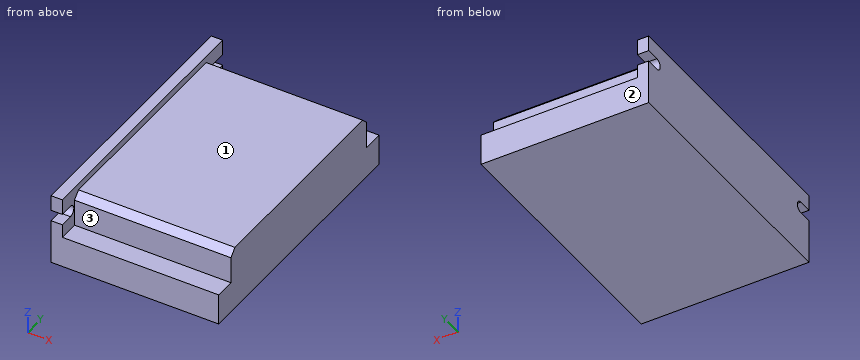
from build123d import *

# Parameters (mm, degrees)
SKETCH_1_W          = 75
SKETCH_1_H          = 100
EXTRUDE_1_DEPTH     = 18
SKETCH_2_W          = 75
SKETCH_2_H          = 118
EXTRUDE_2_DEPTH     = 14
SKETCH_3_W          = 18
SKETCH_3_H          = 118
EXTRUDE_3_DEPTH     = 5
CUT_EXTRUDE_1_DEPTH = 134.529023062
SKETCH_5_W          = 70
SKETCH_5_H          = 100
CUT_EXTRUDE_2_DEPTH = 3
CHAMFER_1_SIZE      = 3


with BuildPart() as part:
    # Эскиз1 → Бобышка-Вытянуть1 (new body)
    with BuildSketch(Plane.XY):
        with Locations((37.5, 50)):
            Rectangle(SKETCH_1_W, SKETCH_1_H)
    extrude(amount=EXTRUDE_1_DEPTH)

    # Эскиз2 → Бобышка-Вытянуть2 (add)
    with BuildSketch(Plane(origin=(0, 0, 0), x_dir=(-1, 0, 0), z_dir=(0, 0, -1))):
        with Locations((-37.5, 50)):
            Rectangle(SKETCH_2_W, SKETCH_2_H)
    extrude(amount=EXTRUDE_2_DEPTH)

    # Эскиз3 → Бобышка-Вытянуть3 (add)
    with BuildSketch(Plane.ZY):
        with Locations((9, 50)):
            Rectangle(SKETCH_3_W, SKETCH_3_H)
    extrude(amount=-EXTRUDE_3_DEPTH)

    # Эскиз4 → Вырез-Вытянуть1 (cut, through all)
    with BuildSketch(Plane.ZY):
        with BuildLine():
            Line((11, 114.734094435), (11, 103))
            ThreePointArc((11, 103), (8.5, 100.5), (6, 103))
            Line((6, 103), (6, 114.734094435))
            ThreePointArc((6, 114.734094435), (8.5, 117.234094435), (11, 114.734094435))
        make_face()
        with BuildLine():
            Line((11, -14.734094435), (11, -3))
            ThreePointArc((11, -3), (8.5, -0.5), (6, -3))
            Line((6, -3), (6, -14.734094435))
            ThreePointArc((6, -14.734094435), (8.5, -17.234094435), (11, -14.734094435))
        make_face()
    extrude(amount=-CUT_EXTRUDE_1_DEPTH, mode=Mode.SUBTRACT)

    # Эскиз5 → Вырез-Вытянуть2 (cut)
    with BuildSketch(Plane.XY.offset(18)):
        with Locations((40, 50)):
            Rectangle(SKETCH_5_W, SKETCH_5_H)
    extrude(amount=-CUT_EXTRUDE_2_DEPTH, mode=Mode.SUBTRACT)

    # Фаска1
    chamfer_1_edges = [part.edges().sort_by_distance(p)[0] for p in [
        (40, 100, 15),
        (40, 0, 15),
    ]]
    chamfer(chamfer_1_edges, length=CHAMFER_1_SIZE)


solid = part.part
Design review of the part built by this model. Coordinates are the model's own, in mm. Face numbers are marked on the shaded views. A direction names the side the tool comes from. Round coordinates to 2 decimals unless told otherwise and drop trailing zeros. Write each loop counter-clockwise with the first axis right and the second up, starting at its lowest first coordinate (ties: lowest second). Pieces come first, ordered by that corner, then holes.
Item 1: Consider section C-C on z = 8.5. Give the boundary of the cut face in (x, y).
Item 2: For the marked faces 1, 2 and 3, list the 3-axis set-ups (+Z, -Z, +X, -X, +Y, -Y) from which the entire face can be reached by the end or side of a thin tool; tool diameter is ignored.
Item 3: For pin 1 Ø21 at (x, y) = (53, 69) entering from +Z; pin 2 Ø7 at (x, y) = (47, -2.5) entering from +Z; pin 3 Ø1 at (x, z) = (25, 3.5) entering from +Y, all flat-tipped, find the tip position at first contact; note any pin that passes through.
Item 4: Consider section B-B on y = 86. Give the boundary of the cut face in (x, z).
Item 5: Wall thickness on L1, parallel to X at y = 45.5, z = 17.5; L2, parallel to Y at x = 44.5, z = 8.5; L3, parallel to Z at x = 69, y = -3: over which ranges is each line inside the solid? List them lowest first.
Item 6: Consider section A-A on x = 57.5. Give the boundary of the cut face in (y, z), and give its area (3 significant figures).
Check values:
1. outline: (0, -0.5) - (5, -0.5) - (5, 0) - (75, 0) - (75, 100) - (5, 100) - (5, 100.5) - (0, 100.5) - close
2. face 1: +Z, +X, +Y, -Y
2. face 2: +Z, -Z, +X, -X, +Y
2. face 3: +Z, +X, -Y
3. pin 1: stops at z = 15
3. pin 2: stops at z = 13
3. pin 3: stops at y = 100
4. outline: (0, -14) - (75, -14) - (75, 15) - (5, 15) - (5, 18) - (0, 18) - close
5. L1: x = 0 to 5
5. L2: y = 0 to 100
5. L3: z = -14 to 0
6. outline: (-9, -14) - (109, -14) - (109, 0) - (100, 0) - (100, 12) - (97, 15) - (3, 15) - (0, 12) - (0, 0) - (-9, 0) - close
6. area: 3,140 mm2
